```python
from build123d import *

# Parameters (mm, degrees)
F0_R     = 35.5
F0_R_2   = 21.5
F1_DEPTH = 12
F2_DEPTH = 520
F3_R     = 35.5
F3_R_2   = 21.5
F4_DEPTH = 10


with BuildPart() as f1:
    # F0 (on Top) → F1 (new body)
    with BuildSketch(Plane.XY):
        with BuildLine():
            Line((75, 181.5), (-75, 181.5))
            ThreePointArc((-75, 181.5), (-96.213203, 172.713203), (-105, 151.5))
            Line((-105, 151.5), (-105, -38.5))
            ThreePointArc((-105, -38.5), (-96.213203, -59.713203), (-75, -68.5))
            Line((-75, -68.5), (75, -68.5))
            ThreePointArc((75, -68.5), (96.213203, -59.713203), (105, -38.5))
            Line((105, -38.5), (105, 151.5))
            ThreePointArc((105, 151.5), (96.213203, 172.713203), (75, 181.5))
        make_face()
        Circle(F0_R, mode=Mode.SUBTRACT)
        Circle(F0_R)
        Circle(F0_R_2, mode=Mode.SUBTRACT)
        Circle(F0_R_2)
    extrude(amount=-F1_DEPTH)

    # F0 (on Top) → F2 (join)
    with BuildSketch(Plane.XY):
        Circle(F0_R)
        Circle(F0_R_2, mode=Mode.SUBTRACT)
    extrude(amount=F2_DEPTH)

    # F3 (on face) → F4 (join)
    with BuildSketch(Plane.XY.offset(520)):
        with BuildLine():
            Line((40, 130), (-40, 130))
            Line((-40, 130), (-40, 0))
            ThreePointArc((-40, 0), (-28.284271, -28.284271), (0, -40))
            ThreePointArc((0, -40), (28.284271, -28.284271), (40, 0))
            Line((40, 0), (40, 130))
        make_face()
        Circle(F3_R, mode=Mode.SUBTRACT)
        Circle(F3_R)
        Circle(F3_R_2, mode=Mode.SUBTRACT)
    extrude(amount=F4_DEPTH)


solid = f1.part
```
CAD build for the part. Positions are in the model's coordinates, mm. A direction names the side the tool comes from. Round coordinates to 2 decimals unless told otherwise and drop trailing zeros. Write each loop counter-clockwise with the first axis right and the second up, starting at its lowest first coordinate (ties: lowest second). Pieces come first, ordered by that corner, then holes.
Item 1: Drill centre lines: L1, parallel to Z at x = 12, y = 108.5; L2, parallel to Y at x = 0, z = 318; L3, parallel to Z at x = 21, y = 131. Where is each one in solid material? Low to high.
Filled in:
L1: z = -12 to 0, 520 to 530
L2: y = -35.5 to -21.5, 21.5 to 35.5
L3: z = -12 to 0
Item 2: Band-saw the part on A-A on y = 13.5. Write the cut outline in (x, z).
Filled in:
outline: (-105, -12) - (105, -12) - (105, 0) - (32.83, 0) - (32.83, 520) - (40, 520) - (40, 530) - (16.73, 530) - (16.73, 0) - (-16.73, 0) - (-16.73, 530) - (-40, 530) - (-40, 520) - (-32.83, 520) - (-32.83, 0) - (-105, 0) - close
Item 3: Tool access for faces 4 (the cylindrical face through (-2.799, 21.317, 261.29)), 5 (the flat face through (40, 64, 525)), 6 (the flat face through (-40, 66, 525)), 7 (the cylindrical face through (-7.696, -34.656, 256.36)), 8 (the flat face through (1, 130, 525)): list every direction of +Z, -Z, +X, -X, +Y, -Y with a clear straight run to the whole face (end or side of a thin tool).
Filled in:
face 4: +Z
face 5: +Z, +X, +Y, -Y
face 6: +Z, -X, +Y, -Y
face 7: none
face 8: +Z, +X, -X, +Y
Item 4: Drop flat-ended pins along their axis: pin 1 Ø21.5 at (x, y) = (8.5, 8.5) entering from +Z; pin 2 Ø4 at (x, z) = (38, 348) entering from +Y; pin 3 Ø11 at (x, z) = (14, 526.5) entering from +Y; pin 4 Ø1 at (x, z) = (-24, 121) entering from +Y. Give the stop position or say it passes through.
Filled in:
pin 1: stops at z = 530
pin 2: passes through
pin 3: stops at y = 130
pin 4: stops at y = 26.61
Item 5: Band-saw the part on B-B on x = 64.5. Write the cut outline in (y, z).
Filled in:
outline: (-68.5, -12) - (181.5, -12) - (181.5, 0) - (-68.5, 0) - close
Item 6: Band-saw the part on C-C on z = 462. Write the cut outline in (x, y), then the cut area to 3 significant figures.
Filled in:
outline: circle Ø71 at (0, 0); hole circle Ø43 at (0, 0)
area: 2,510 mm2
Item 7: Mould opens along X. For faces 1 (the flat face through (0, 0, 0)), 2 (the flat face through (105, 55, -6)), 3 (the flat face through (-1, 58, -12)) say: released by +X, released by -X, zero draft, split by the parting line, or undercut.
Filled in:
face 1: undercut
face 2: released by +X
face 3: zero draft
